Autodesk Inventor part; units mm, degrees
ref_plane "YZ Plane" through (0, 0, 0) normal (1, 0, 0) x (0, 1, 0)
ref_plane "XZ Plane" through (0, 0, 0) normal (0, 1, 0) x (-1, 0, 0)
ref_plane "XY Plane" through (0, 0, 0) normal (0, 0, 1) x (1, 0, 0)
sketch "Skizze1" plane through (0, 0, 0) normal (0, 0, 1) x (1, 0, 0)
  line L0 (-24, 0) -> (144, 0)
  line L1 (0, -27.6) -> (0, 165.6)
  line L2 (0, 0) -> (120, 0)
  line L3 (120, 0) -> (120, 138)
  line L4 (120, 138) -> (0, 138)
  line L5 (0, 138) -> (0, 0)
  point P0 (0, 138)
  dimension "d0" = 120
  dimension "d1" = 138
extrude "Extrusion1" add sketch "Skizze1" along normal blind 8
sketch "Skizze2" plane through (0, 0, 0) normal (0, 0, -1) x (-1, 0, 0)
  line L0 (-75, 118) -> (-70, 118)
  line L1 (-70, 118) -> (-70, 113)
  line L2 (-70, 113) -> (-75, 113)
  line L3 (-75, 113) -> (-75, 118)
  line L4 (-50, 118) -> (-45, 118)
  line L5 (-45, 118) -> (-45, 113)
  line L6 (-45, 113) -> (-50, 113)
  line L7 (-50, 113) -> (-50, 118)
  line L8 (0, 138) -> (0, 0)
  line L9 (-120, 0) -> (-120, 138)
  line L10 (-120, 138) -> (0, 138)
  dimension "d4" = 5
  dimension "d5" = 5
  dimension "d6" = 5
  dimension "d7" = 5
  dimension "d8" = 45
  dimension "d9" = 45
  dimension "d10" = 20
  dimension "d11" = 20
extrude "Extrusion2" add sketch "Skizze2" along normal blind 20
sketch "Skizze3" plane through (0, 0, -20) normal (0, 0, -1) x (-1, 0, 0)
  line L0 (-70, 118) -> (-75, 118)
  line L1 (-70, 113) -> (-70, 118)
  line L2 (-75, 118) -> (-70, 118)
  line L3 (-70, 118) -> (-70, 113)
  line L4 (-70, 113) -> (-75, 113)
  line L5 (-75, 113) -> (-75, 118)
  point P0 (0, 0)
extrude "Extrusion3" add sketch "Skizze3" along normal blind 5
sketch "Skizze4" plane through (70, 113, 0) normal (-1, 0, 0) x (0, 0, 1)
  line L0 (0, 5) -> (-25, 5)
  line L1 (-20, 5) -> (-20, 0)
  line L2 (-25, 5) -> (-20, 5)
  line L3 (-20, 5) -> (-20, 0)
  line L4 (-20, 0) -> (-25, 0)
  line L5 (-25, 0) -> (-25, 5)
  point P0 (0, -113)
extrude "Extrusion4" add sketch "Skizze4" along normal blind 25
fillet "Rundung1" radius 2.5 12 edges at (70, 113, -10) (75, 113, -12.5) (60, 113, -20) (60, 113, -25) (50, 113, -10) (45, 113, -12.5) (60, 118, -25) (70, 118, -10) (75, 118, -12.5) (60, 118, -20) (45, 118, -12.5) (50, 118, -10)
sketch "Skizze7" plane through (0, 0, 0) normal (0, 0, -1) x (-1, 0, 0)
  point P0 (0, 0)
sketch "Skizze8" plane through (0, 0, 0) normal (0, 0, -1) x (-1, 0, 0)
  line L0 (-120, 0) -> (-120, 138)
  line L1 (0, 138) -> (0, 0)
  line L2 (-120, 5) -> (0, 5)
  line L3 (0, 5) -> (0, 0)
  line L4 (0, 0) -> (-120, 0)
  line L5 (-120, 0) -> (-120, 5)
  point P0 (0, 5)
  dimension "d25" = 5
extrude "Extrusion7" cut sketch "Skizze8" against normal blind 10
properties part number "DeckelMess" material "Acetalharz, Schwarz"
Could you check a few things on this model? Use its own coordinates, in mm. Give positions to 0.01 mm unless a question says otherwise; leave off trailing zeros. Write each loop counter-clockwise with the first axis right and the second up, starting at its lowest first coordinate (ties: lowest second). Pieces come first, ordered by that corner, then holes. Notation, with made-up numbers: (-7.75, -1.75) - (36.25, -1.75) arc R28 cw to (36.25, 19.25) - close; hole circle Ø6 at (-19, 42.5). An arc over 180 degrees is marked (long way). Use CSV: the item, a comma, the result in double quotes. Start each with the question number.
Item 1: If I drill on line 1 along Z through (x, y) = (80, 118); line 2 along Y through (x, z) = (61.5, -22), over which ranges is the centre line in solid material (lowest first)?
Item 2: I'm going to push flat-ended pins straight in: pin 1 (5 mm diameter, centred on x = 79.5, y = 85, fed in from -Z); pin 2 (3 mm diameter, centred on x = 74.5, z = -3.5, fed in from +Y). Where does each tip first touch, or does it pass through?
Item 3: I want a section at D-D, the plane y = 122. Please give me the cut outline in (x, z).
Item 4: I want a section at C-C, the plane x = 28.5. Please give me the cut outline in (y, z), then the cut area to 3 significant figures.
Findings:
1,line 1,"z = 0 to 8"
1,line 2,"y = 113.05 to 117.95"
2,pin 1,"stops at z = 0"
2,pin 2,"stops at y = 117.95"
3,outline,"(0, 0) - (120, 0) - (120, 8) - (0, 8) - close"
4,outline,"(5, 0) - (138, 0) - (138, 8) - (5, 8) - close"
4,area,"1,060 mm2"
